```python
from build123d import *

# Parameters (mm, degrees)
F0_W     = 463
F0_H     = 693
F0_W_2   = 460
F0_H_2   = 690
F1_DEPTH = 355
F3_DEPTH = 463.001


with BuildPart() as f1:
    # F0 (on Top) → F1 (new body)
    with BuildSketch(Plane.XY):
        Rectangle(F0_W, F0_H)
        Rectangle(F0_W_2, F0_H_2, mode=Mode.SUBTRACT)
    extrude(amount=-F1_DEPTH)

    # F2 (on face) → F3 (cut, through all)
    with BuildSketch(Plane.YZ.offset(231.5)):
        Polygon((346.5, -355), (-346.5, -2), (-346.5, -355), align=None)
    extrude(amount=-F3_DEPTH, mode=Mode.SUBTRACT)


solid = f1.part
```
The listing builds one solid part. Answer for the finished solid, in the listing's coordinates (mm). Round coordinates to 2 decimals unless told otherwise and drop trailing zeros. Loops run counter-clockwise (first coordinate to the right, second up) from the corner with the lowest first, then second, coordinate; pieces in that order, holes last. Notation, with made-up numbers: (20, 15) - (45, 15) arc R6 ccw to (45, 26) - close; hole circle Ø8 at (73, -10). An arc over 180 degrees is marked (long way). Return JSON: item names as keys, results as strings. Group by question number.
1. The part is cut by section A-A on x = 52. Determine the outline of the cut face in (y, z), then the cut area to 4 significant figures.
2. Consider probe 1 along X at (y, z) = (-53, -74.5); probe 2 along Y at (x, z) = (-74.5, -86). Determine where each line is inside the solid, lowest interval first.
3. The mould has two halves that part along X. Classify faces 1 (the flat face through (-3, 346.5, -175)), 2 (the flat face through (230, 72, -135)), 3 (the flat face through (231.5, 72, -136)), 4 (the flat face through (-231.5, 72, -136)): pulls with the +X half, pulls with the -X half, needs draft (parallel to the pull), parting line crosses it, or undercut.
4. The part is cut by section C-C on z = -118. Determine the outline of the cut face in (x, y).
5. The part is cut by section D-D on z = -271. Determine the outline of the cut face in (x, y), then the cut area to 3 significant figures.
6. The part is cut by section B-B on y = -229.5. Determine the outline of the cut face in (x, z).
7. This flat-tipped pin is pushed along its axis until it touches: P1, Ø6, axis at x = -113.5, z = -156, coming from the -Y side. Where does it stop, or does it pass through?
Resolved:
{
 "1": {"outline": "(-346.5, -2) - (-345, -2.76) - (-345, 0) - (-346.5, 0) - close; (345, -354.24) - (346.5, -355) - (346.5, 0) - (345, 0) - close", "area": "535.5 mm²"},
 "2": {"probe 1": "x = -231.5 to -230, 230 to 231.5", "probe 2": "y = 345 to 346.5"},
 "3": {"face 1": "needs draft", "face 2": "undercut", "face 3": "pulls with the +X half", "face 4": "pulls with the -X half"},
 "4": {"outline": "(-231.5, -118.77) - (-230, -118.77) - (-230, 345) - (230, 345) - (230, -118.77) - (231.5, -118.77) - (231.5, 346.5) - (-231.5, 346.5) - close"},
 "5": {"outline": "(-231.5, 181.59) - (-230, 181.59) - (-230, 345) - (230, 345) - (230, 181.59) - (231.5, 181.59) - (231.5, 346.5) - (-231.5, 346.5) - close", "area": "1,180 mm²"},
 "6": {"outline": "(-231.5, -61.6) - (-230, -61.6) - (-230, 0) - (-231.5, 0) - close; (230, -61.6) - (231.5, -61.6) - (231.5, 0) - (230, 0) - close"},
 "7": {"P1": "stops at y = 345"}
}
